Part model, mm, in its own coordinate system. Face numbers are marked on the shaded views. A direction names the side the tool comes from. Give positions to 0.01 mm unless a question says otherwise; leave off trailing zeros. Write each loop counter-clockwise with the first axis right and the second up, starting at its lowest first coordinate (ties: lowest second). Pieces come first, ordered by that corner, then holes. Notation, with made-up numbers: M -18,19 L -8,19 A22 ccw -8,46 Z; hole C 77,32.25 d3. An arc over 180 degrees is marked long. Use CSV: the item, a comma, the result in double quotes. Start each with the question number.
1. Drop flat-ended pins along their axis: pin 1 Ø10 at (x, y) = (37.5, -65) entering from -Z; pin 2 Ø1.5 at (x, z) = (23, -20) entering from -Y; pin 3 Ø7.5 at (x, y) = (10, -8.5) entering from +Z; pin 4 Ø5 at (x, z) = (-43, -28) entering from -Y. Give the stop position or say it passes through.
2. Band-saw the part on C-C, the plane x = -43. List the corners of the cut face in (y, z).
3. Band-saw the part on B-B, the plane z = 28. List the corners of the cut face in (x, y), then the cut area to 3 significant figures.
4. Drill centre lines: line 1 along X through (y, z) = (1.2, -28); line 2 along X through (y, z) = (-53, 0); line 3 along Z through (x, y) = (-18, -22). Where is each one in solid material? Low to high. Write a range as from..to.
5. Mould opens along X. For the marked faces 1, 2 and 3 say: pulls with the +X half, pulls with the -X half, needs draft (parallel to the pull), parting line crosses it, or undercut.
6. 3-axis set-ups, long thin cutter, end or side, ignore diameter. For the marked faces 4, 5 and 6: which of +Z, -Z, +X, -X, +Y, -Y reach the whole face in a straight line?
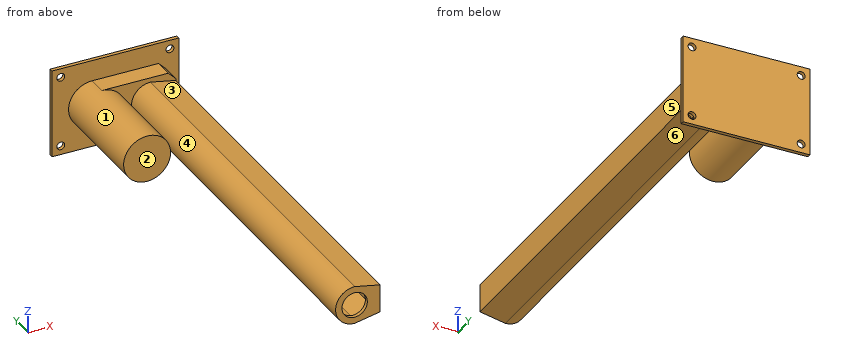
from build123d import *

# Parameters (mm, degrees)
SKETCH_1_W                  = 100
SKETCH_1_H                  = 70
EXTRUDE_1_DEPTH             = 3
SKETCH_2_R                  = 3.1
CUT_EXTRUDE_1_DEPTH         = 62.10646447
PATTERN_LINEAR_2_COUNT      = 2
PATTERN_LINEAR_2_PITCH      = 56
PATTERN_LINEAR_2_COUNT_DIR2 = 2
PATTERN_LINEAR_2_PITCH_DIR2 = 86
EXTRUDE_2_DEPTH             = 15
CHAMFER_2_SIZE              = 6
SKETCH_4_R                  = 18.5
EXTRUDE_3_DEPTH             = 70
EXTRUDE_4_DEPTH             = 315
SHELL_START                 = -327
SHELL_5_DEPTH               = 327
SHELL_START_2               = -82
SHELL_5_2_OUTLINE_R         = 15.5
SHELL_5_2_DEPTH             = 82
SHELL_START_3               = -12
SHELL_5_3_DEPTH             = 12
CUT_EXTRUDE_2_REACH         = 340.547
SKETCH_6_R                  = 10


# Read off the part's stored shape, not the designer's step: 抽壳5
with BuildPart() as part:
    # 草图1 → 凸台-拉伸1 (new body)
    with BuildSketch(Plane(origin=(0, 0, 0), x_dir=(1, 0, 0), z_dir=(0, 1, 0))):
        Rectangle(SKETCH_1_W, SKETCH_1_H)
    extrude(amount=EXTRUDE_1_DEPTH)

    # 草图2 → 切除-拉伸1 (cut, through all)
    with BuildSketch(Plane(origin=(0, 3, 0), x_dir=(1, 0, 0), z_dir=(0, 1, 0))):
        with Locations(Location((-43, 28, 0), (0, 0, 270))):
            Circle(SKETCH_2_R)
    cut_extrude_1 = extrude(amount=-CUT_EXTRUDE_1_DEPTH, mode=Mode.SUBTRACT)

    # 阵列(线性)2: Cut-Extrude 1 2 × 2
    with Locations(*[(j * PATTERN_LINEAR_2_PITCH_DIR2, 0, i * PATTERN_LINEAR_2_PITCH) for i in range(PATTERN_LINEAR_2_COUNT) for j in range(PATTERN_LINEAR_2_COUNT_DIR2) if (i, j) != (0, 0)]):
        add(cut_extrude_1, mode=Mode.SUBTRACT)

    # 草图3 → 凸台-拉伸2 (add)
    with BuildSketch(Plane.XZ):
        with BuildLine():
            Line((-18.4, 18.5), (40, 18.5))
            Line((40, 18.5), (40, -18.5))
            Line((40, -18.5), (-18.4, -18.5))
            ThreePointArc((-18.4, -18.5), (-36.9, 0), (-18.4, 18.5))
        make_face()
    extrude(amount=EXTRUDE_2_DEPTH)

    # 倒角2
    chamfer_2_edges = [part.edges().sort_by_distance(p)[0] for p in [
        (40, -7.5, -18.5),
        (40, -7.5, 18.5),
    ]]
    chamfer(chamfer_2_edges, length=CHAMFER_2_SIZE)

    # 草图4 → 凸台-拉伸3 (add)
    with BuildSketch(Plane(origin=(0, -15, 0), x_dir=(-1, 0, 0), z_dir=(0, -1, 0))):
        with Locations(Location((18.4, 0, 0), (0, 0, 90))):
            Circle(SKETCH_4_R)
    extrude(amount=EXTRUDE_3_DEPTH)

    # 草图5 → 凸台-拉伸4 (add)
    with BuildSketch(Plane.XZ.offset(15)):
        with BuildLine():
            ThreePointArc((20, -15), (5, 0), (20, 15))
            Line((20, 15), (20, -15))
        make_face()
        Polygon((20, -15), (40, -11), (40, 11), (20, 15), align=None)
    extrude(amount=EXTRUDE_4_DEPTH)

    # 抽壳5 outline → 抽壳5 (cut)
    with BuildSketch(Plane(origin=(0, 0, 0), x_dir=(1, 0, 0), z_dir=(0, 1, 0)).offset(SHELL_START)):
        with BuildLine():
            Line((37, -8.540588292), (37, 8.540588292))
            Line((37, 8.540588292), (19.719352649, 11.996717762))
            ThreePointArc((19.719352649, 11.996717762), (8, 0), (19.719352649, -11.996717762))
            Line((19.719352649, -11.996717762), (37, -8.540588292))
        make_face()
    extrude(amount=SHELL_5_DEPTH, mode=Mode.SUBTRACT)

    # Shell 5 2 outline → Shell 5 2 (cut)
    with BuildSketch(Plane(origin=(0, 0, 0), x_dir=(1, 0, 0), z_dir=(0, 1, 0)).offset(SHELL_START_2)):
        with Locations((-18.4, 0)):
            Circle(SHELL_5_2_OUTLINE_R)
    extrude(amount=SHELL_5_2_DEPTH, mode=Mode.SUBTRACT)

    # Shell 5 3 outline → Shell 5 3 (cut)
    with BuildSketch(Plane(origin=(0, 0, 0), x_dir=(1, 0, 0), z_dir=(0, 1, 0)).offset(SHELL_START_3)):
        with BuildLine():
            Line((32.757359313, 15.5), (-18.4, 15.5))
            ThreePointArc((-18.4, 15.5), (-2.9, 0), (-18.4, -15.5))
            Line((-18.4, -15.5), (32.757359313, -15.5))
            Line((32.757359313, -15.5), (37, -11.257359313))
            Line((37, -11.257359313), (37, -8.540588292))
            Line((37, -8.540588292), (19.719352649, -11.996717762))
            ThreePointArc((19.719352649, -11.996717762), (8, 0), (19.719352649, 11.996717762))
            Line((19.719352649, 11.996717762), (37, 8.540588292))
            Line((37, 8.540588292), (37, 11.257359313))
            Line((37, 11.257359313), (32.757359313, 15.5))
        make_face()
    extrude(amount=SHELL_5_3_DEPTH, mode=Mode.SUBTRACT)

    # 草图6 → 切除-拉伸2 (cut, up to next)
    with BuildSketch(Plane.XZ.offset(330), mode=Mode.PRIVATE) as cut_extrude_2_sk1:
        with Locations(Location((20, 0, 0), (0, 0, 270))):
            Circle(SKETCH_6_R)
    cut_extrude_2_tool1 = extrude(cut_extrude_2_sk1.sketch, amount=-CUT_EXTRUDE_2_REACH, mode=Mode.PRIVATE) & part.part
    add(cut_extrude_2_tool1.solids().sort_by_distance((20, -330, 0))[0], mode=Mode.SUBTRACT)


solid = part.part
Output:
1,pin 1,"stops at z = -12.5"
1,pin 2,"stops at y = 0"
1,pin 3,"stops at z = 18.5"
1,pin 4,"passes through"
2,outline,"M 0,-35 L 3,-35 L 3,-31.1 L 0,-31.1 Z; M 0,-24.9 L 3,-24.9 L 3,24.9 L 0,24.9 Z; M 0,31.1 L 3,31.1 L 3,35 L 0,35 Z"
3,outline,"M -50,0 L -46.1,0 L -46.1,3 L -50,3 Z; M -39.9,0 L 39.9,0 L 39.9,3 L -39.9,3 Z; M 46.1,0 L 50,0 L 50,3 L 46.1,3 Z"
3,area,"263 mm²"
4,line 1,"x = -50..-46.1, -39.9..39.9, 46.1..50"
4,line 2,"x = -36.9..-33.9, -2.9..0.1, 5..8, 37..40"
4,line 3,"z = -18.5..-15.49, 15.49..18.5"
5,face 1,"undercut"
5,face 2,"needs draft"
5,face 3,"pulls with the +X half"
6,face 4,"-Y"
6,face 5,"+Z, -Z, +X, -Y"
6,face 6,"-Z, +X, -Y"
